Part print with two shaded views. Sizes in mm from the minimum x, y, z corner. A direction names the side the tool comes from. Coordinates: 2 decimals unless noted, no trailing zeros. Loops run counter-clockwise (first coordinate to the right, second up) from the corner with the lowest first, then second, coordinate; pieces in that order, holes last. Notation, with made-up numbers: (-5, 65.25) -> (34, 65.25) arc R27 cw to (34, 101.25) -> close; hole circle Ø4 at (60, -21). An arc over 180 degrees is marked (long way). Return JSON: item names as keys, results as strings. Group by question number.
(1) Tool access for the marked faces 1 and 2: list every direction of +Z, -Z, +X, -X, +Y, -Y with a clear straight run to the whole face (end or side of a thin tool).
(2) Saw through at D-D on x = 18. Write the cut outline in (y, z).
(3) Mould opens along X. For the marked faces 3 and 4 say: pulls with the +X half, pulls with the -X half, needs draft (parallel to the pull), parting line crosses it, or undercut.
(4) Saw through at C-C on y = 20. Write the cut outline in (x, z), then the cut area to 3 significant figures.
(5) Saw through at B-B on x = 36.5. Write the cut outline in (y, z).
(6) Probe L1, parallel to Y at x = 36.5, z = 6.4; L2, parallel to Y at x = 36.5, z = 12.5; L3, parallel to X at y = 39.5, z = 6.25. List the from-to ranges inside material, lowest first.
(7) Flat gauge pins, fed straight in: pin 1 Ø2.5 at (x, y) = (3.6, 36.5) entering from +Z; pin 2 Ø3 at (x, z) = (47.5, 6.5) entering from +Y; pin 3 Ø1.2 at (y, z) = (6.5, 12.5) entering from +X; pin 4 Ø8 at (y, z) = (20.5, 12) entering from +X. Where does each tip first touch, or does it go through?
(8) Saw through at A-A on z = 12. Write the cut outline in (x, y).
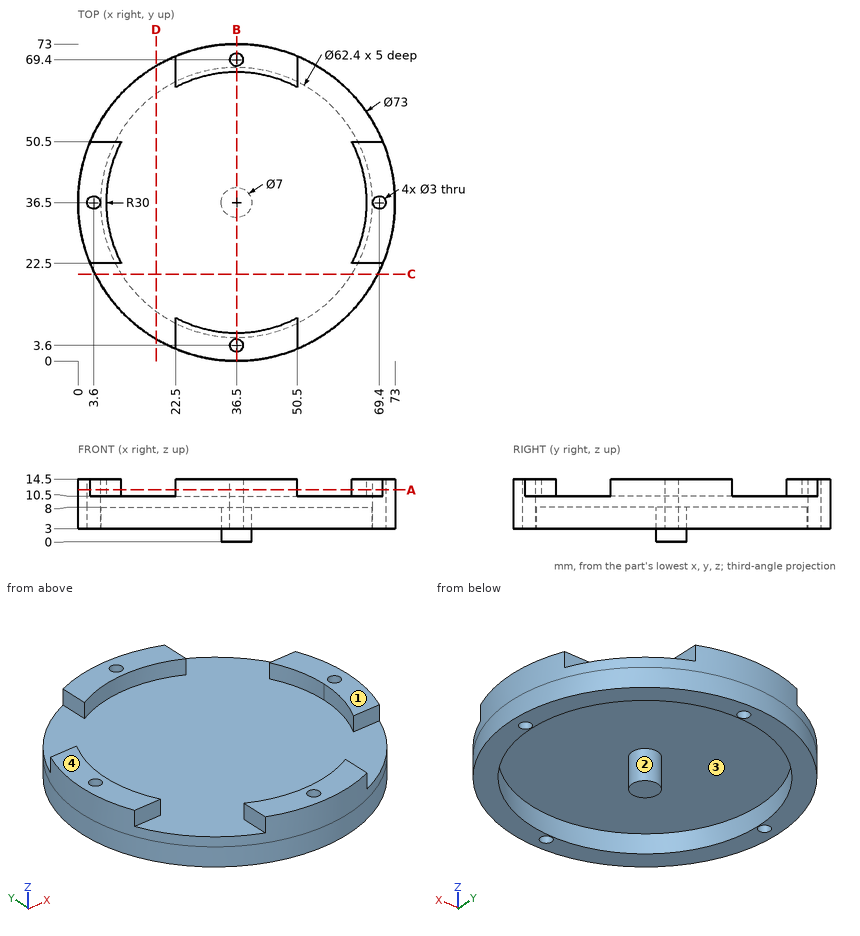
Geometry results:
{
 "1": {"face 1": "+Z, +X, -X, +Y, -Y", "face 2": "-Z"},
 "2": {"outline": "(5.04, 3) -> (11.38, 3) -> (11.38, 8) -> (61.62, 8) -> (61.62, 3) -> (67.96, 3) -> (67.96, 10.5) -> (5.04, 10.5) -> close"},
 "3": {"face 3": "undercut", "face 4": "needs draft"},
 "4": {"outline": "(3.94, 3) -> (10.02, 3) -> (10.02, 8) -> (62.98, 8) -> (62.98, 3) -> (69.06, 3) -> (69.06, 10.5) -> (3.94, 10.5) -> close", "area": "224 mm²"},
 "5": {"outline": "(0, 3) -> (2.1, 3) -> (2.1, 14.5) -> (0, 14.5) -> close; (5.1, 3) -> (5.3, 3) -> (5.3, 8) -> (33, 8) -> (33, 0) -> (40, 0) -> (40, 8) -> (67.7, 8) -> (67.7, 3) -> (67.9, 3) -> (67.9, 14.5) -> (66.5, 14.5) -> (66.5, 10.5) -> (6.5, 10.5) -> (6.5, 14.5) -> (5.1, 14.5) -> close; (70.9, 3) -> (73, 3) -> (73, 14.5) -> (70.9, 14.5) -> close"},
 "6": {"L1": "0 to 2.1, 5.1 to 5.3, 33 to 40, 67.7 to 67.9, 70.9 to 73", "L2": "0 to 2.1, 5.1 to 6.5, 66.5 to 67.9, 70.9 to 73", "L3": "0.12 to 5.44, 34.7 to 38.3, 67.56 to 72.88"},
 "7": {"pin 1": "through", "pin 2": "y = 71.74", "pin 3": "x = 50.5", "pin 4": "x = 70.97"},
 "8": {"outline": "(2.79, 22.5) -> (9.97, 22.5) arc R30 cw to (9.97, 50.5) -> (2.79, 50.5) arc R36.5 ccw to start; (22.5, 2.79) arc R36.5 ccw to (50.5, 2.79) -> (50.5, 9.97) arc R30 cw to (22.5, 9.97) -> close; (22.5, 63.03) arc R30 cw to (50.5, 63.03) -> (50.5, 70.21) arc R36.5 ccw to (22.5, 70.21) -> close; (63.03, 22.5) -> (70.21, 22.5) arc R36.5 ccw to (70.21, 50.5) -> (63.03, 50.5) arc R30 cw to start; hole circle Ø3 at (3.6, 36.5); hole circle Ø3 at (36.5, 3.6); hole circle Ø3 at (36.5, 69.4); hole circle Ø3 at (69.4, 36.5)"}
}
